Here's how the part is built. I have some questions about the finished solid (model axes, mm). Round coordinates to 2 decimals unless told otherwise and drop trailing zeros. One line per item, written item: value. Start each with the question number.
Item 1: If I drill on line 1 (Y direction, x = 441, z = 22.5), over which ranges is the centre line in solid material (lowest first)?
Item 2: Imagine slicing it at A-A, the plane x = -439.5. Count the separate pieces of the cut face and the enclosed holes in it, then the cut area to 3 significant figures.
Item 3: For P1, Ø2, axis at x = 411.5, y = -51, coming from the -Z side; P2, Ø1, axis at x = 296, z = 75.5, coming from the -Y side; P3, Ø0.5, axis at x = 119, y = -54.5, coming from the +Z side, each with a flat end and sliding along its axis, tell me the tip position at first contact or that it passes through.
```python
from build123d import *

# Parameters (mm, degrees)
F1_DEPTH      = 641.35
F2_R          = 31.75
F3_DEPTH      = 641.35
F3_DEPTH_BACK = 641.35
F4_R          = 1.27
F5_DEPTH      = 1282.701


# Not quite as in the source:
# - ends of sketch curves that miss each other by under 0.0002 mm in the source are joined


with BuildPart() as f1:
    # F0 (on Right) → F1 (new body, symmetric)
    with BuildSketch(Plane.YZ):
        Polygon((-1.27, 0), (0, 0), (0, 57.15), (-1.27, 57.15), (-1.27, 52.07), align=None)
    extrude(amount=F1_DEPTH, both=True)

    # F2 (on Right) → F3 (join, two sides)
    with BuildSketch(Plane.YZ) as f3_sk:
        with Locations((-31.75, 57.15)):
            Circle(F2_R)
    extrude(amount=F3_DEPTH)
    extrude(f3_sk.sketch, amount=-F3_DEPTH_BACK)

    # F4 (on face) → F5 (cut, through all)
    with BuildSketch(Plane.YZ.offset(641.35)):
        with BuildLine():
            ThreePointArc((-62.2299973542, 57.1373), (-31.7436499999, 26.6700006615), (-1.27, 57.15))
            ThreePointArc((-1.27, 57.15), (-31.7436499999, 87.6299993385), (-62.2299973542, 57.1627))
            Line((-62.2299973542, 57.1627), (-61.5949972979, 57.1627))
            ThreePointArc((-61.5949972979, 57.1627), (-31.7436499999, 86.9949993245), (-1.905, 57.15))
            ThreePointArc((-1.905, 57.15), (-31.7436499999, 27.3050006755), (-61.5949972979, 57.1373))
            Line((-61.5949972979, 57.1373), (-62.2299973542, 57.1373))
        make_face()
        with BuildLine():
            ThreePointArc((-3.175, 57.15), (-31.7436499998, 85.7249992944), (-60.3249971778, 57.1627))
            Line((-60.3249971778, 57.1627), (-59.6899971136, 57.1627))
            ThreePointArc((-59.6899971136, 57.1627), (-31.7436499998, 85.0899992784), (-3.81, 57.15))
            ThreePointArc((-3.81, 57.15), (-31.7436499998, 29.2100007216), (-59.6899971136, 57.1373))
            Line((-59.6899971136, 57.1373), (-60.3249971778, 57.1373))
            ThreePointArc((-60.3249971778, 57.1373), (-31.7436499998, 28.5750007056), (-3.175, 57.15))
        make_face()
        with BuildLine():
            ThreePointArc((-5.08, 57.15), (-31.7436499998, 83.819999244), (-58.4199969762, 57.1627))
            Line((-58.4199969762, 57.1627), (-57.7849969024, 57.1627))
            ThreePointArc((-57.7849969024, 57.1627), (-31.7436499998, 83.1849992256), (-5.715, 57.15))
            ThreePointArc((-5.715, 57.15), (-31.7436499998, 31.1150007744), (-57.7849969024, 57.1373))
            Line((-57.7849969024, 57.1373), (-58.4199969762, 57.1373))
            ThreePointArc((-58.4199969762, 57.1373), (-31.7436499998, 30.480000756), (-5.08, 57.15))
        make_face()
        with BuildLine():
            ThreePointArc((-6.985, 57.15), (-31.7436499998, 81.9149991859), (-56.5149967436, 57.1626999999))
            Line((-56.5149967436, 57.1626999999), (-55.8799969024, 57.1627))
            ThreePointArc((-55.8799969024, 57.1627), (-31.7436499998, 81.279999409), (-7.6199997555, 57.15))
            ThreePointArc((-7.6199997555, 57.15), (-31.7436499998, 33.020000591), (-55.8799969024, 57.1373))
            Line((-55.8799969024, 57.1373), (-56.5149969762, 57.1373))
            ThreePointArc((-56.5149969762, 57.1373), (-31.7436499998, 32.3850008141), (-6.985, 57.15))
        make_face()
        with BuildLine():
            ThreePointArc((-8.8899997286, 57.15), (-31.7436499998, 80.0099993894), (-54.6099967436, 57.1626999999))
            Line((-54.6099967436, 57.1626999999), (-53.9749969024, 57.1627))
            ThreePointArc((-53.9749969024, 57.1627), (-31.7436499997, 79.3749996239), (-9.524999469, 57.15))
            ThreePointArc((-9.524999469, 57.15), (-31.7436499997, 34.9250003761), (-53.9749969024, 57.1373))
            Line((-53.9749969024, 57.1373), (-54.6099969762, 57.1373))
            ThreePointArc((-54.6099969762, 57.1373), (-31.7436499998, 34.2900006106), (-8.8899997286, 57.15))
        make_face()
        with BuildLine():
            ThreePointArc((-10.7949994079, 57.15), (-31.7436499997, 78.10499963), (-52.7049967436, 57.1626999999))
            Line((-52.7049967436, 57.1626999999), (-52.0699969024, 57.1627))
            ThreePointArc((-52.0699969024, 57.1627), (-31.7436499997, 77.469999879), (-11.4299991288, 57.15))
            ThreePointArc((-11.4299991288, 57.15), (-31.7436499997, 36.830000121), (-52.0699969024, 57.1373))
            Line((-52.0699969024, 57.1373), (-52.7049969762, 57.1373))
            ThreePointArc((-52.7049969762, 57.1373), (-31.7436499997, 36.19500037), (-10.7949994079, 57.15))
        make_face()
        with BuildLine():
            ThreePointArc((-12.6999987905, 57.15), (-31.7436499996, 76.2000001512), (-50.7999969762, 57.1627000001))
            Line((-50.7999969762, 57.1627), (-50.1649969024, 57.1627))
            ThreePointArc((-50.1649969024, 57.1627), (-31.7436499996, 75.5650001869), (-13.3349987183, 57.15))
            ThreePointArc((-13.3349987183, 57.15), (-31.7436499996, 38.7349998131), (-50.1649969024, 57.1373))
            Line((-50.1649969024, 57.1373), (-50.7999969762, 57.1373))
            ThreePointArc((-50.7999969762, 57.1372999999), (-31.7436499996, 38.0999998488), (-12.6999987905, 57.15))
        make_face()
        with BuildLine():
            ThreePointArc((-14.6049985527, 57.15), (-31.7436499996, 74.2950002714), (-48.8949967436, 57.1626999999))
            Line((-48.8949967436, 57.1626999999), (-48.2599969024, 57.1627))
            ThreePointArc((-48.2599969024, 57.1627), (-31.7436499995, 73.6600005659), (-15.2399982129, 57.15))
            ThreePointArc((-15.2399982129, 57.15), (-31.7436499995, 40.6399994341), (-48.2599969024, 57.1373))
            Line((-48.2599969024, 57.1373), (-48.8949969762, 57.1373))
            ThreePointArc((-48.8949969762, 57.1373), (-31.7436499996, 40.0049997286), (-14.6049985527, 57.15))
        make_face()
        with BuildLine():
            ThreePointArc((-16.5099979647, 57.15), (-31.7436499995, 72.3900007123), (-46.9899967436, 57.1626999999))
            Line((-46.9899967436, 57.1626999999), (-46.3549969024, 57.1627))
            ThreePointArc((-46.3549969024, 57.1627), (-31.7436499994, 71.7550010437), (-17.1449975758, 57.15))
            ThreePointArc((-17.1449975758, 57.15), (-31.7436499994, 42.5449989563), (-46.3549969024, 57.1373))
            Line((-46.3549969024, 57.1373), (-46.9899969762, 57.1373))
            ThreePointArc((-46.9899969762, 57.1373), (-31.7436499995, 41.9099992877), (-16.5099979647, 57.15))
        make_face()
        with BuildLine():
            ThreePointArc((-18.4149972088, 57.15), (-31.7436499993, 70.4850012793), (-45.0849967436, 57.1626999999))
            Line((-45.0849967436, 57.1626999999), (-44.4499969024, 57.1627))
            ThreePointArc((-44.4499969024, 57.1627), (-31.7436499992, 69.8500016649), (-19.0499967476, 57.15))
            ThreePointArc((-19.0499967476, 57.15), (-31.7436499992, 44.4499983351), (-44.4499969024, 57.1373))
            Line((-44.4499969024, 57.1373), (-45.0849969762, 57.1373))
            ThreePointArc((-45.0849969762, 57.1373), (-31.7436499993, 43.8149987207), (-18.4149972088, 57.15))
        make_face()
        with BuildLine():
            ThreePointArc((-20.3199959683, 57.15), (-31.743649999, 68.5800022679), (-43.1799969762, 57.1627000001))
            Line((-43.1799969762, 57.1627), (-42.5449969024, 57.1627))
            ThreePointArc((-42.5449969024, 57.1627), (-31.7436499989, 67.9450025054), (-20.954995627, 57.15))
            ThreePointArc((-20.954995627, 57.15), (-31.7436499989, 46.3549974946), (-42.5449969024, 57.1373))
            Line((-42.5449969024, 57.1373), (-43.1799969762, 57.1373))
            ThreePointArc((-43.1799969762, 57.1372999999), (-31.743649999, 45.7199977321), (-20.3199959683, 57.15))
        make_face()
        with BuildLine():
            ThreePointArc((-22.2249947897, 57.15), (-31.7436499987, 66.6750030936), (-41.2749967436, 57.1626999998))
            Line((-41.2749967436, 57.1626999998), (-40.6399969024, 57.1627))
            ThreePointArc((-40.6399969024, 57.1627), (-31.7436499984, 66.040003706), (-22.8599940261, 57.15))
            ThreePointArc((-22.8599940261, 57.15), (-31.7436499984, 48.259996294), (-40.6399969024, 57.1373))
            Line((-40.6399969024, 57.1373), (-41.2749969762, 57.1373))
            ThreePointArc((-41.2749969762, 57.1373), (-31.7436499987, 47.6249969064), (-22.2249947897, 57.15))
        make_face()
        with BuildLine():
            ThreePointArc((-24.1299926731, 57.15), (-31.7436499979, 64.7700046811), (-39.3699967436, 57.1626999998))
            Line((-39.3699967436, 57.1626999998), (-38.7349969024, 57.1627))
            ThreePointArc((-38.7349969024, 57.1627), (-31.7436499974, 64.1350055615), (-24.7649915521, 57.15))
            ThreePointArc((-24.7649915521, 57.15), (-31.7436499974, 50.1649944385), (-38.7349969024, 57.1373))
            Line((-38.7349969024, 57.1373), (-39.3699969762, 57.1373))
            ThreePointArc((-39.3699969762, 57.1373), (-31.7436499979, 49.5299953189), (-24.1299926731, 57.15))
        make_face()
        with BuildLine():
            ThreePointArc((-26.0349891453, 57.15), (-31.7436499962, 62.8650073269), (-37.4649967436, 57.1626999997))
            Line((-37.4649967436, 57.1626999997), (-36.8299969024, 57.1627))
            ThreePointArc((-36.8299969024, 57.1627), (-31.743649995, 62.2300088087), (-26.6699872226, 57.15))
            ThreePointArc((-26.6699872226, 57.15), (-31.743649995, 52.0699911913), (-36.8299969024, 57.1373))
            Line((-36.8299969024, 57.1373), (-37.4649969762, 57.1373))
            ThreePointArc((-37.4649969762, 57.1373), (-31.7436499962, 51.4349926731), (-26.0349891453, 57.15))
        make_face()
        with Locations((-31.75, 57.15)):
            Circle(F4_R)
    extrude(amount=-F5_DEPTH, mode=Mode.SUBTRACT)


solid = f1.part
```
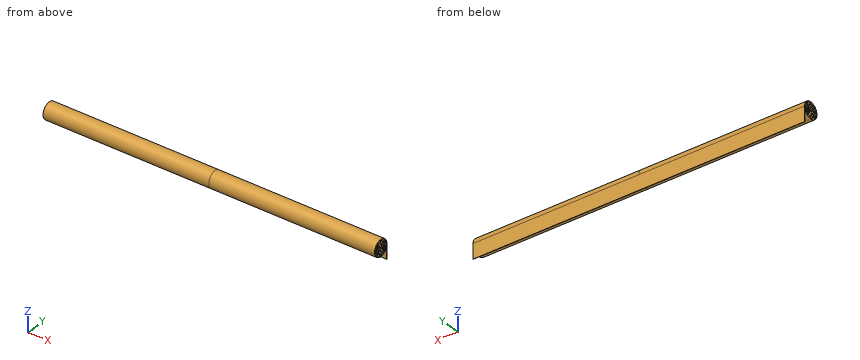
Values follow:
1. line 1: y = -1.27 to 0
2. separate pieces: 1
2. enclosed holes: 15
2. area: 2,230 mm^2
3. P1: stops at z = 31.17
3. P2: stops at y = -58.01
3. P3: stops at z = 79.55
